Verification items for the finished model (mm, model axes). Face numbers are marked on the shaded views. A direction names the side the tool comes from. Give positions to 0.01 mm unless a question says otherwise; leave off trailing zeros. Order: outer loops, then holes, each group sorted by start corner. A loop starts at its lowest first (then second) coordinate and runs counter-clockwise, first axis right, second up. Notation, with made-up numbers: (34.25, 66) -> (61.25, 66) arc R25 ccw to (61.25, 87) -> close; hole circle Ø2 at (-34, 65). An arc over 180 degrees is marked (long way). One line per question, with ' | ' between items. Start each with the question number.
Q1. Section check C-C on z = -18.9. Record the cut outline in (x, y).
Q2. Material ranges on probe 1 along X at (y, z) = (2.2, -5.5); probe 2 along Z at (x, y) = (0, 2.2); probe 3 along Z at (x, y) = (-30, 2), recorded low to high. Write a range as [from, to].
Q3. Access from +Z, -Z, +X, -X, +Y, -Y to the whole of each face (thin tool, end or side, straight path). Record for the marked faces 5 and 6.
Q4. Section check D-D on y = 2.9. Give the number of separate pieces and of enclosed holes in the cut face, plus the area to 3 significant figures.
Q5. Go/stop test with flat-tipped pins: pin 1 (0.8 mm diameter, centred on y = 1.5, z = -17.5, fed in from -X); pin 2 (1.2 mm diameter, centred on x = -47.5, y = 3, fed in from +Z). Record where each tip stops, or that it passes through.
Q6. Section check A-A on x = -30. Record the cut outline in (y, z), plus the area to 3 significant figures.
Q7. Mould release check, pull along Z, two halves, no side actions. Record for the marked faces 1, 2, 3 and 4: released by +Z, released by -Z, zero draft, split by the parting line, or undercut.
Q8. Section check B-B on x = -12. Record the cut outline in (y, z), plus the area to 3 significant figures.
Autodesk Inventor part; units mm, degrees
ref_plane "YZ Plane" through (0, 0, 0) normal (1, 0, 0) x (0, 1, 0)
ref_plane "XZ Plane" through (0, 0, 0) normal (0, 1, 0) x (-1, 0, 0)
ref_plane "XY Plane" through (0, 0, 0) normal (0, 0, 1) x (1, 0, 0)
sketch "Sketch1" plane through (0, 0, 0) normal (0, 1, 0) x (-1, 0, 0)
  line L0 (0, 0) -> (60, 0)
  line L1 (60, 0) -> (60, -10)
  line L2 (60, -10) -> (0, -10)
  line L3 (0, -10) -> (0, 0)
  circle A0 centre (60, 0) radius 1.5
  circle A1 centre (60, -10) radius 1.5
  circle A2 centre (0, 0) radius 1.5
  circle A3 centre (0, -10) radius 1.5
  line L4 (60, -10) -> (63, -10)
  line L5 (63, -10) -> (63, -13)
  line L6 (63, -13) -> (60, -13)
  line L7 (60, -13) -> (60, -10)
  line L8 (0, 0) -> (-3, 0)
  line L9 (-3, 0) -> (-3, 3)
  line L10 (-3, 3) -> (0, 3)
  line L11 (0, 3) -> (0, 0)
  line L12 (-3, 3) -> (63, 3)
  line L13 (63, 3) -> (63, -13)
  line L14 (63, -13) -> (-3, -13)
  line L15 (-3, -13) -> (-3, 3)
  line L16 (60, -5) -> (0, -5)
  line L17 (24, 7) -> (36, 7)
  line L18 (36, 7) -> (36, -17)
  line L19 (36, -17) -> (24, -17)
  line L20 (24, -17) -> (24, 7)
  line L21 (24, 7) -> (36, -17) construction
  line L22 (36, 7) -> (24, -17) construction
  line L23 (30, -5) -> (30, 6.25)
  line L24 (30, 6.25) -> (30, 8.9)
  circle A4 centre (30, 8.9) radius 1
  line L25 (30, -5) -> (30, -16.25)
  line L26 (30, -16.25) -> (30, -18.9)
  circle A5 centre (30, -18.9) radius 1
  line L27 (36, 7) -> (24, 7)
  line L28 (24, 7) -> (24, 11)
  line L29 (24, 11) -> (36, 11)
  line L30 (36, 11) -> (36, 7)
  line L31 (36, -17) -> (24, -17)
  line L32 (24, -17) -> (24, -21)
  line L33 (24, -21) -> (36, -21)
  line L34 (36, -21) -> (36, -17)
  line L35 (36, 11) -> (38, 11)
  line L36 (38, 11) -> (38, -21)
  line L37 (38, -21) -> (36, -21)
  line L38 (36, -21) -> (36, 11)
  line L39 (24, 11) -> (20.9428, 11)
  line L40 (24, 9) -> (24, 11)
  line L41 (24, 11) -> (22, 11)
  line L42 (22, 11) -> (22, -21)
  line L43 (22, -21) -> (24, -21)
  line L44 (24, -21) -> (24, 11)
  line L45 (60, -5) -> (55, -5)
  line L46 (55, -5) -> (40, -5)
  line L47 (40, -5) -> (40, 0)
  line L48 (40, 0) -> (55, 0)
  line L49 (55, 0) -> (55, -5)
  line L50 (55, 0) -> (40, 0)
  line L51 (40, 0) -> (40, -10)
  line L52 (40, -10) -> (55, -10)
  line L53 (55, -10) -> (55, 0)
  line L54 (0, -5) -> (5, -5)
  line L55 (5, -5) -> (20, -5)
  line L56 (20, -5) -> (20, 0)
  line L57 (20, 0) -> (5, 0)
  line L58 (5, 0) -> (5, -5)
  line L59 (20, 0) -> (5, 0)
  line L60 (5, 0) -> (5, -10)
  line L61 (5, -10) -> (20, -10)
  line L62 (20, -10) -> (20, 0)
  point P0 (24, -13)
  point P1 (24, 3)
  point P2 (38, 3)
  point P3 (38, -13)
  point P4 (22, -13)
  point P5 (22, 3)
  dimension "d0" = 60
  dimension "d1" = 10
  dimension "d2" = 3
  dimension "d3" = 3
  dimension "d4" = 3
  dimension "d5" = 3
  dimension "d6" = 3
  dimension "d7" = 3
  dimension "d8" = 3
  dimension "d9" = 3
  dimension "d12" = 12
  dimension "d13" = 24
  dimension "d14" = 11.25
  dimension "d15" = 2.65
  dimension "d16" = 2
  dimension "d17" = 11.25
  dimension "d18" = 2.65
  dimension "d19" = 2
  dimension "d20" = 4
  dimension "d21" = 4
  dimension "d22" = 2
  dimension "d24" = 2
  dimension "d28" = 5
  dimension "d29" = 15
  dimension "d30" = 5
  dimension "d31" = 5
  dimension "d32" = 15
extrude "Extrusion1" add sketch "Sketch1" along normal blind 4 contours A2 L11 L12 L42 L0 | L0 L58 L16 L3 A2 | L3 A3 L2 L42 L14 L15 L8 A2 | L8 L9 L10 L11 A2 | L16 L60 L2 A3 L3 | L0 L42 L16 L56 | L42 L39 L28 L20 L12 | L12 L20 L0 L42 | L0 L20 L16 L42 | L16 L42 L2 L62 | L42 L2 L20 L14 | L14 L20 L32 L43 L42 | L16 L20 L2 L42 | L28 L29 L30 L17 | L19 L34 L33 L32 | L18 L30 L35 L36 L12 | L12 L36 L0 L18 | L0 L36 L16 L18 | L18 L2 L36 L14 | L14 L36 L37 L34 L18 | L12 L13 L4 A1 L1 A0 L0 L36 | L0 L47 L16 L36 | L16 L36 L2 L18 | L36 L2 A1 L7 L14 | L16 L51 L2 L36 | L7 A1 L4 L5 L6 | L0 A0 L1 L16 L49 | L16 L1 A1 L2 L53
fillet "Fillet1" radius 4 4 edges at (-22, 2, 3) (-22, 2, -13) (-38, 2, -13) (-38, 2, 3)
fillet "Fillet2" radius 3 4 edges at (-38, 2, 11) (-22, 2, 11) (-22, 2, -21) (-38, 2, -21)
fillet "Fillet3" radius 3 4 edges at (-63, 2, 3) (-63, 2, -13) (3, 2, -13) (3, 2, 3)
fillet "Fillet4" radius 2 8 edges at (-55, 2, -10) (-40, 2, -10) (-40, 2, 0) (-55, 2, 0) (-20, 2, -10) (-20, 2, 0) (-5, 2, 0) (-5, 2, -10)
properties part number "microservo_support1"
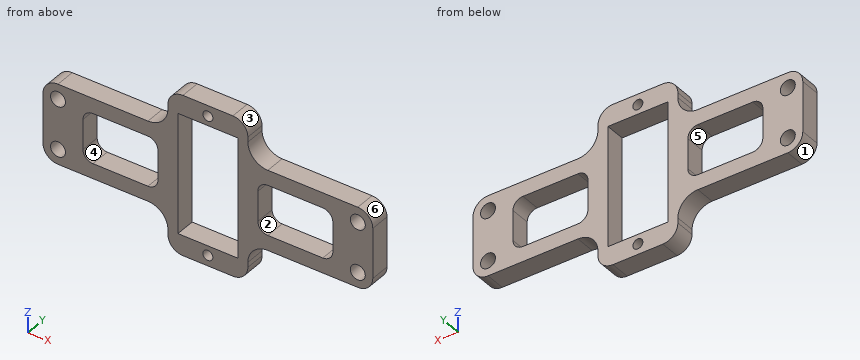
Filled in:
1) outline: (-37.86, 0) -> (-31, 0) -> (-31, 4) -> (-37.86, 4) -> close; (-29, 0) -> (-22.14, 0) -> (-22.14, 4) -> (-29, 4) -> close
2) probe 1: [-63, -55], [-40, -36], [-24, -20], [-5, 3] | probe 2: [-13, -11.5], [-8.5, -1.5], [1.5, 3] | probe 3: [-21, -19.9], [-17.9, -17], [7, 7.9], [9.9, 11]
3) face 5: +Y, -Y | face 6: +Z, +X, +Y, -Y
4) separate pieces: 1 | enclosed holes: 9 | area: 695 mm²
5) pin 1: x = -38 | pin 2: z = 3
6) outline: (0, -21) -> (4, -21) -> (4, -19.9) -> (0, -19.9) -> close; (0, -17.9) -> (4, -17.9) -> (4, -17) -> (0, -17) -> close; (0, 7) -> (4, 7) -> (4, 7.9) -> (0, 7.9) -> close; (0, 9.9) -> (4, 9.9) -> (4, 11) -> (0, 11) -> close | area: 16.0 mm²
7) face 1: released by -Z | face 2: undercut | face 3: released by +Z | face 4: undercut
8) outline: (0, -13) -> (4, -13) -> (4, -10) -> (0, -10) -> close; (0, 0) -> (4, 0) -> (4, 3) -> (0, 3) -> close | area: 24.0 mm²
